from build123d import *

# Parameters (mm, degrees)
ESQUISSE1_W             = 20
ESQUISSE1_H             = 3
ESQUISSE1_H_2           = 4
BOSS_EXTRU_1_DEPTH      = 3
ESQUISSE2_W             = 172
ESQUISSE2_H             = 1
ENL_V_MAT_EXTRU_1_DEPTH = 1.5
ESQUISSE4_W             = 3
ESQUISSE4_H             = 20
ENL_V_MAT_EXTRU_2_DEPTH = 207.455986147


with BuildPart() as part:
    # Esquisse1 → Boss.-Extru.1 (new body)
    with BuildSketch(Plane.XY):
        with BuildLine():
            Line((-109.499197329, 0), (62.500802671, 0))
            Line((62.500802671, 0), (62.500802671, -175))
            Line((62.500802671, -175), (56.500802671, -175))
            ThreePointArc((56.500802671, -175), (-23.499197329, -130.484780132), (-103.499197329, -175))
            Line((-103.499197329, -175), (-109.499197329, -175))
            Line((-109.499197329, -175), (-109.499197329, 0))
        make_face()
        with Locations((-83.499197329, -123.5)):
            Rectangle(ESQUISSE1_W, ESQUISSE1_H, mode=Mode.SUBTRACT)
        with Locations((-23.499197329, -124)):
            Rectangle(ESQUISSE1_W, ESQUISSE1_H_2, mode=Mode.SUBTRACT)
        with Locations((36.500802671, -123.5)):
            Rectangle(ESQUISSE1_W, ESQUISSE1_H, mode=Mode.SUBTRACT)
    extrude(amount=BOSS_EXTRU_1_DEPTH)

    # Esquisse2 → Enlèv. mat.-Extru.1 (cut)
    with BuildSketch(Plane.XY.offset(3)):
        with Locations((-23.499197329, -1)):
            Rectangle(ESQUISSE2_W, ESQUISSE2_H)
    extrude(amount=-ENL_V_MAT_EXTRU_1_DEPTH, mode=Mode.SUBTRACT)

    # Esquisse4 → Enlèv. mat.-Extru.2 (cut, through all)
    with BuildSketch(Plane.XY.offset(3)):
        with Locations((-107.999197329, -78.25)):
            Rectangle(ESQUISSE4_W, ESQUISSE4_H)
        with Locations((61.000802671, -78.25)):
            Rectangle(ESQUISSE4_W, ESQUISSE4_H)
    extrude(amount=-ENL_V_MAT_EXTRU_2_DEPTH, mode=Mode.SUBTRACT)


solid = part.part
Here's how the part is built. I have some questions about the finished solid (model axes, mm). Coordinates: 2 decimals unless noted, no trailing zeros. Loops run counter-clockwise (first coordinate to the right, second up) from the corner with the lowest first, then second, coordinate; pieces in that order, holes last. Notation, with made-up numbers: (-38, -34.5) -> (-1, -34.5) arc R12 ccw to (-1, -11.5) -> close; hole circle Ø1 at (78.5, -9). An arc over 180 degrees is marked (long way). Use one line per item in the form item = value. Start each with the question number.
(1) If we section it at A-A (x = -23.5): Please give me the cut outline in (y, z), then the cut area to 3 significant figures.
(2) If we section it at C-C (x = -2): Please give me the cut outline in (y, z), then the cut area to 3 significant figures.
(3) If we section it at D-D (x = -81.5): Please give me the cut outline in (y, z), then the cut area to 3 significant figures.
(4) Will these pins go through, and if not, where does the flat tip stop? pin 1 (0.9 mm diameter, centred on x = -85.5, z = 1, fed in from -Y); pin 2 (1.5 mm diameter, centred on x = 41, z = 2, fed in from -Y); pin 3 (0.5 mm diameter, centred on x = -52.5, y = -1, fed in from +Z).
(5) Please list where these lines run through material, in increasing order: line 1 along Y through (x, z) = (39, 2.75); line 2 along Y through (x, z) = (44.5, 1.8); line 3 along X through (y, z) = (-158.5, 2.65).
(6) If we section it at B-B (z = 2.1): Give the number of separate pieces and of enclosed holes in the cut face, then the cut area to 3 significant figures.
Verdict:
q1.outline = (-130.48, 0) -> (-126, 0) -> (-126, 3) -> (-130.48, 3) -> close; (-122, 0) -> (0, 0) -> (0, 3) -> (-0.5, 3) -> (-0.5, 1.5) -> (-1.5, 1.5) -> (-1.5, 3) -> (-122, 3) -> close
q1.area = 378 mm²
q2.outline = (-132.97, 0) -> (0, 0) -> (0, 3) -> (-0.5, 3) -> (-0.5, 1.5) -> (-1.5, 1.5) -> (-1.5, 3) -> (-132.97, 3) -> close
q2.area = 397 mm²
q3.outline = (-150.47, 0) -> (-125, 0) -> (-125, 3) -> (-150.47, 3) -> close; (-122, 0) -> (0, 0) -> (0, 3) -> (-0.5, 3) -> (-0.5, 1.5) -> (-1.5, 1.5) -> (-1.5, 3) -> (-122, 3) -> close
q3.area = 441 mm²
q4.pin_1 = -154.18
q4.pin_2 = -156.76
q4.pin_3 = 1.5
q5.line_1 = -154.22 to -125, -122 to -1.5, -0.5 to 0
q5.line_2 = -159.52 to -125, -122 to -1.5, -0.5 to 0
q5.line_3 = -109.5 to -90.51, 43.51 to 62.5
q6.separate_pieces = 2
q6.enclosed_holes = 3
q6.area = 24,600 mm²
